```python
from build123d import *

# Parameters (mm, degrees)
M14X1_5_TAPPED_HOLE1_D              = 12.5
M14X1_5_TAPPED_HOLE1_DEPTH          = 25.4
M14X1_5_TAPPED_HOLE1_TIP            = 3.755378869
F_1_16_0_0625_DIAMETER_HOLE1_D      = 1.5875
F_1_16_0_0625_DIAMETER_HOLE1_DEPTH  = 28.575
F_1_16_0_0625_DIAMETER_HOLE1_TIP    = 0.476933116
F_3_32_0_09375_DIAMETER_HOLE1_D     = 2.38125
F_3_32_0_09375_DIAMETER_HOLE1_DEPTH = 28.702
F_3_32_0_09375_DIAMETER_HOLE1_TIP   = 0.715399675
F_1_4_0_25_DIAMETER_HOLE1_D         = 6.35
CIRPATTERN1_COUNT                   = 6
F_1_32_0_03125_DIAMETER_HOLE2_D     = 0.79375
F_1_32_0_03125_DIAMETER_HOLE2_DEPTH = 28.575
F_1_32_0_03125_DIAMETER_HOLE2_TIP   = 0.238466558


with BuildPart() as part:
    # Sketch1 → Revolve1 (revolve)
    with BuildSketch(Plane.XY):
        Polygon((-6.35, 0), (-31.75, 0), (-31.75, 38.1), (-3.81, 38.1), (-3.81, 6.35), (-6.35, 6.35), align=None)
    revolve(axis=Axis((0, 0, 0), (0, 1, 0)))

    # M14x1.5 Tapped Hole1
    with Locations(Plane(origin=(0, 38.1, 0), x_dir=(1, 0, 0), z_dir=(0, 1, 0))):
        with Locations((0, 0)):
            Hole(M14X1_5_TAPPED_HOLE1_D / 2, depth=M14X1_5_TAPPED_HOLE1_DEPTH)
            with Locations((0, 0, -(M14X1_5_TAPPED_HOLE1_DEPTH + M14X1_5_TAPPED_HOLE1_TIP / 2))):  # 118° drill point
                Cone(0, M14X1_5_TAPPED_HOLE1_D / 2, M14X1_5_TAPPED_HOLE1_TIP, mode=Mode.SUBTRACT)

    # Sketch6 → 1/4 NPT Tapped Hole1 (revolve, cut)
    with BuildSketch(Plane(origin=(31.75, 19.05, 0), x_dir=(0, 0, -1), z_dir=(0, 1, 0))):
        Polygon((0, 0), (0, 20.360347279), (5.5626, 17.018), (5.5626, 9.906), (5.943685794, 9.906), (6.2402847, 0), align=None)
    revolve(axis=Axis((38.1, 19.05, 0), (-1, 0, 0)), mode=Mode.SUBTRACT)

    # Sketch8 → 1/4 NPT Tapped Hole2 (revolve, cut)
    with BuildSketch(Plane(origin=(-31.75, 19.05, 0), x_dir=(0, 0, 1), z_dir=(0, 1, 0))):
        Polygon((0, 0), (0, 20.360347279), (5.5626, 17.018), (5.5626, 9.906), (5.943685794, 9.906), (6.2402847, 0), align=None)
    revolve(axis=Axis((-38.1, 19.05, 0), (1, 0, 0)), mode=Mode.SUBTRACT)

    # 1/16 (0.0625) Diameter Hole1
    with Locations(Plane(origin=(31.75, 0, 0), x_dir=(0, 0, -1), z_dir=(1, 0, 0))):
        with Locations((0, 19.05)):
            Hole(F_1_16_0_0625_DIAMETER_HOLE1_D / 2, depth=F_1_16_0_0625_DIAMETER_HOLE1_DEPTH)
            with Locations((0, 0, -(F_1_16_0_0625_DIAMETER_HOLE1_DEPTH + F_1_16_0_0625_DIAMETER_HOLE1_TIP / 2))):  # 118° drill point
                Cone(0, F_1_16_0_0625_DIAMETER_HOLE1_D / 2, F_1_16_0_0625_DIAMETER_HOLE1_TIP, mode=Mode.SUBTRACT)

    # 3/32 (0.09375) Diameter Hole1
    with Locations(Plane.ZY.offset(31.75)):
        with Locations((0, 19.05)):
            Hole(F_3_32_0_09375_DIAMETER_HOLE1_D / 2, depth=F_3_32_0_09375_DIAMETER_HOLE1_DEPTH)
            with Locations((0, 0, -(F_3_32_0_09375_DIAMETER_HOLE1_DEPTH + F_3_32_0_09375_DIAMETER_HOLE1_TIP / 2))):  # 118° drill point
                Cone(0, F_3_32_0_09375_DIAMETER_HOLE1_D / 2, F_3_32_0_09375_DIAMETER_HOLE1_TIP, mode=Mode.SUBTRACT)

    # 1/4 (0.25) Diameter Hole1 (through all)
    with Locations(Plane(origin=(0, 38.1, 0), x_dir=(1, 0, 0), z_dir=(0, 1, 0))):
        with Locations((21.997045256, 12.7)):
            f_1_4_0_25_diameter_hole1 = Hole(F_1_4_0_25_DIAMETER_HOLE1_D / 2)

    # CirPattern1: 1/4 (0.25) Diameter Hole1 ×6 about axis
    cirpattern1_axis = Axis((0, 0, 0), (0, 1, 0))
    for i in range(1, CIRPATTERN1_COUNT):
        add(f_1_4_0_25_diameter_hole1.rotate(cirpattern1_axis, i * 360 / CIRPATTERN1_COUNT), mode=Mode.SUBTRACT)

    # Sketch18 → 1/4 NPT Tapped Hole3 (revolve, cut)
    with BuildSketch(Plane(origin=(-15.875, 19.05, 27.49630657), x_dir=(0.866025404, 0, 0.5), z_dir=(0, 1, 0))):
        Polygon((0, 0), (0, 19.344347279), (5.5626, 16.002), (5.5626, 9.906), (5.943685794, 9.906), (6.2402847, 0), align=None)
    revolve(axis=Axis((-19.05, 19.05, 32.995567884), (0.5, 0, -0.866025404)), mode=Mode.SUBTRACT)

    # 1/32 (0.03125) Diameter Hole2
    with Locations(Plane(origin=(-15.875, 0, 27.49630657), x_dir=(0, -1, 0), z_dir=(-0.5, 0, 0.866025404))):
        with Locations((-19.05, 0)):
            Hole(F_1_32_0_03125_DIAMETER_HOLE2_D / 2, depth=F_1_32_0_03125_DIAMETER_HOLE2_DEPTH)
            with Locations((0, 0, -(F_1_32_0_03125_DIAMETER_HOLE2_DEPTH + F_1_32_0_03125_DIAMETER_HOLE2_TIP / 2))):  # 118° drill point
                Cone(0, F_1_32_0_03125_DIAMETER_HOLE2_D / 2, F_1_32_0_03125_DIAMETER_HOLE2_TIP, mode=Mode.SUBTRACT)


solid = part.part
```
Read the model definition and answer for the solid it produces. Units are mm, in the model's axes. A direction names the side the tool comes from. Coordinates: 2 decimals unless noted, no trailing zeros. Write each loop counter-clockwise with the first axis right and the second up, starting at its lowest first coordinate (ties: lowest second). Pieces come first, ordered by that corner, then holes. Notation, with made-up numbers: (65.25, -22.75) -> (92.25, -22.75) arc R23 ccw to (92.25, -8.75) -> close; hole circle Ø3 at (78, 31). An arc over 180 degrees is marked (long way). Return JSON: item names as keys, results as strings.
1. Find the intervals of material crossed by line 1 along Z through (x, y) = (0, 8.6) (3 decimals); line 2 along Y through (x, z) = (-9, 16); line 3 along Z through (x, y) = (0, 27) (3 decimals), in increasing order. Write a range as from..to.
Found:
{"line 1": "-31.75..-28.575, -22.225..-3.81, 3.81..22.225, 28.575..31.75", "line 2": "0..13.49, 24.61..38.1", "line 3": "-31.75..-28.575, -22.225..-6.25, 6.25..22.225, 28.575..31.75"}
2. A cutting plane is placed at A-A (x = 0). Determine the outline of the cut face in (y, z) (3 decimals), and give its area (3 significant figures).
Found:
{"outline": "(0, -31.75) -> (38.1, -31.75) -> (38.1, -28.575) -> (0, -28.575) -> close; (0, -22.225) -> (38.1, -22.225) -> (38.1, -6.25) -> (12.7, -6.25) -> (11.234, -3.81) -> (6.35, -3.81) -> (6.35, -6.35) -> (0, -6.35) -> close; (0, 6.35) -> (6.35, 6.35) -> (6.35, 3.81) -> (11.234, 3.81) -> (12.7, 6.25) -> (38.1, 6.25) -> (38.1, 22.225) -> (0, 22.225) -> close; (0, 28.575) -> (38.1, 28.575) -> (38.1, 31.75) -> (0, 31.75) -> close", "area": "1,490 mm2"}
3. Determine the mould class of faces 1 (the face through (19.064, 18.783, -11.484)), 2 (the face through (-14.65, 19.32, -28.17)), 3 (the face through (-26.87, 18.78, -6.09)) for opening direction X: pulls with the +X half, pulls with the -X half, needs draft (parallel to the pull), parting line crosses it, or undercut.
Found:
{"face 1": "undercut", "face 2": "parting line crosses it", "face 3": "pulls with the -X half"}
4. A cutting plane is placed at C-C (x = -24). Determine the outline of the cut face in (y, z), and give its area (3 significant figures).
Found:
{"outline": "(0, -20.79) -> (38.1, -20.79) -> (38.1, -15.16) -> (0, -15.16) -> close; (0, -10.24) -> (38.1, -10.24) -> (38.1, 10.24) -> (0, 10.24) -> close; (0, 15.16) -> (38.1, 15.16) -> (38.1, 20.79) -> (0, 20.79) -> close; hole circle Ø12.02 at (19.05, 0)", "area": "1,100 mm2"}
5. Each of these flat-tipped pins is pushed along its axis until it touches: P1, Ø4, axis at x = 0, z = -25.4, coming from the -Y side; P2, Ø10, axis at y = 19.05, z = 0, coming from the -X side; P3, Ø3, axis at x = -19, y = 5.5, coming from the -Z side; P4, Ø3.5, axis at y = 18.5, z = 1.5, coming from the +X side. Where does it stop, or does it pass through?
Found:
{"P1": "through", "P2": "x = -14.39", "P3": "z = -26.49", "P4": "x = 13.4"}
6. A cutting plane is placed at B-B (z = -25.4). Determine the outline of the cut face in (x, y) (3 decimals).
Found:
{"outline": "(-19.05, 0) -> (-3.175, 0) -> (-3.175, 38.1) -> (-19.05, 38.1) -> close; (3.175, 0) -> (19.05, 0) -> (19.05, 38.1) -> (3.175, 38.1) -> close"}
7. A tool of negligible diameter and unlimited length cuts with its end or side. For faces 4 (the face through (-6.55, 19.75, 11.04)), 5 (the face through (-21.844, 21.2, -5.3)), 6 (the face through (26.87, 18.78, 6.09)), from which of +Z, -Z, +X, -X, +Y, -Y can it reach the whole face along a straight path? Write none if from no direction.
Found:
{"face 4": "none", "face 5": "-X", "face 6": "+X"}
8. A cutting plane is placed at D-D (z = -12.7). Determine the outline of the cut face in (x, y).
Found:
{"outline": "(-29.1, 0) -> (-25.17, 0) -> (-25.17, 38.1) -> (-29.1, 38.1) -> close; (-18.82, 0) -> (18.82, 0) -> (18.82, 38.1) -> (-18.82, 38.1) -> close; (25.17, 0) -> (29.1, 0) -> (29.1, 38.1) -> (25.17, 38.1) -> close"}
